Verification items for the finished model (mm, model axes). Face numbers are marked on the shaded views. A direction names the side the tool comes from. Give positions to 0.01 mm unless a question says otherwise; leave off trailing zeros. Loops run counter-clockwise (first coordinate to the right, second up) from the corner with the lowest first, then second, coordinate; pieces in that order, holes last. Notation, with made-up numbers: M 56,7.25 L 67,7.25 A19 cw 67,19.25 Z; hole C 28.25,19.5 d5. An arc over 180 degrees is marked long. Write each question's results on one line, items separated by ' | '. Start each with the question number.
```python
from build123d import *

# Parameters (mm, degrees)
SKETCH1_W           = 50
SKETCH1_H           = 52
BOSS_EXTRUDE1_DEPTH = 61
SKETCH2_W           = 30
SKETCH2_H           = 30
CUT_EXTRUDE1_DEPTH  = 51
CUT_EXTRUDE2_DEPTH  = 75
CUT_EXTRUDE3_DEPTH  = 51
SKETCH6_W           = 50
SKETCH6_H           = 4.1
BOSS_EXTRUDE2_DEPTH = 43
SKETCH8_R           = 11.5
SKETCH8_R_2         = 2
CUT_EXTRUDE4_DEPTH  = 43
BOSS_EXTRUDE3_DEPTH = 3.5
BOSS_EXTRUDE4_DEPTH = 3.5
SKETCH11_R          = 15
CUT_EXTRUDE5_DEPTH  = 98.5
SKETCH12_R          = 15
CUT_EXTRUDE6_DEPTH  = 98.5


with BuildPart() as part:
    # Sketch1 → Boss-Extrude1 (new body)
    with BuildSketch(Plane(origin=(0, 0, 0), x_dir=(1, 0, 0), z_dir=(0, 1, 0))):
        Rectangle(SKETCH1_W, SKETCH1_H)
    extrude(amount=BOSS_EXTRUDE1_DEPTH)

    # Sketch2 → Cut-Extrude1 (cut)
    with BuildSketch(Plane(origin=(0, 61, 0), x_dir=(1, 0, 0), z_dir=(0, 1, 0))):
        Rectangle(SKETCH2_W, SKETCH2_H)
    extrude(amount=-CUT_EXTRUDE1_DEPTH, mode=Mode.SUBTRACT)

    # Sketch3 → Cut-Extrude2 (cut, symmetric)
    with BuildSketch(Plane(origin=(0, 10, 0), x_dir=(1, 0, 0), z_dir=(0, 1, 0))):
        with BuildLine():
            Line((1, 12.5), (1, -12.5))
            ThreePointArc((1, -12.5), (-2, -15.5), (-5, -12.5))
            Line((-5, -12.5), (-5, 12.5))
            ThreePointArc((-5, 12.5), (-2, 15.5), (1, 12.5))
        make_face()
    extrude(amount=CUT_EXTRUDE2_DEPTH, both=True, mode=Mode.SUBTRACT)

    # Sketch5 → Cut-Extrude3 (cut)
    with BuildSketch(Plane(origin=(0, 61, 0), x_dir=(1, 0, 0), z_dir=(0, 1, 0))):
        with BuildLine():
            Line((3.852906206, 15), (3.852906206, -15))
            ThreePointArc((3.852906206, -15), (-2.147093794, -21), (-8.147093794, -15))
            Line((-8.147093794, -15), (-8.147093794, 15))
            ThreePointArc((-8.147093794, 15), (-2.147093794, 21), (3.852906206, 15))
        make_face()
    extrude(amount=-CUT_EXTRUDE3_DEPTH, mode=Mode.SUBTRACT)

    # Sketch6 → Boss-Extrude2 (add)
    with BuildSketch(Plane(origin=(0, 61, 0), x_dir=(1, 0, 0), z_dir=(0, 1, 0))):
        with Locations((0, 23.95)):
            Rectangle(SKETCH6_W, SKETCH6_H)
    extrude(amount=BOSS_EXTRUDE2_DEPTH)

    # Sketch8 → Cut-Extrude4 (cut)
    with BuildSketch(Plane.XY.offset(-21.9)):
        with Locations((-0.305876732, 83.277637399)):
            Circle(SKETCH8_R)
        with Locations((-15.355876732, 68.327637399)):
            Circle(SKETCH8_R_2)
        with Locations((-15.355876732, 98.327637399)):
            Circle(SKETCH8_R_2)
        with Locations((14.644123268, 68.327637399)):
            Circle(SKETCH8_R_2)
        with Locations((14.644123268, 98.327637399)):
            Circle(SKETCH8_R_2)
    extrude(amount=-CUT_EXTRUDE4_DEPTH, mode=Mode.SUBTRACT)

    # Sketch9 → Boss-Extrude3 (add)
    with BuildSketch(Plane.ZY.offset(25)):
        Polygon((-21.9, 61), (2.05, 61), (-21.9, 82.893920103), align=None)
    extrude(amount=-BOSS_EXTRUDE3_DEPTH)

    # Sketch10 → Boss-Extrude4 (add)
    with BuildSketch(Plane(origin=(25, 0, 0), x_dir=(0, 0, -1), z_dir=(1, 0, 0))):
        Polygon((21.9, 61), (-2.05, 61), (21.9, 82.893920103), align=None)
    extrude(amount=-BOSS_EXTRUDE4_DEPTH)

    # Sketch11 → Cut-Extrude5 (cut)
    with BuildSketch(Plane.XY.offset(26)):
        with Locations((0, 36)):
            Circle(SKETCH11_R)
    extrude(amount=-CUT_EXTRUDE5_DEPTH, mode=Mode.SUBTRACT)

    # Sketch12 → Cut-Extrude6 (cut)
    with BuildSketch(Plane(origin=(25, 0, 0), x_dir=(0, 0, -1), z_dir=(1, 0, 0))):
        with Locations((-2.05, 36)):
            Circle(SKETCH12_R)
    extrude(amount=-CUT_EXTRUDE6_DEPTH, mode=Mode.SUBTRACT)


solid = part.part
```
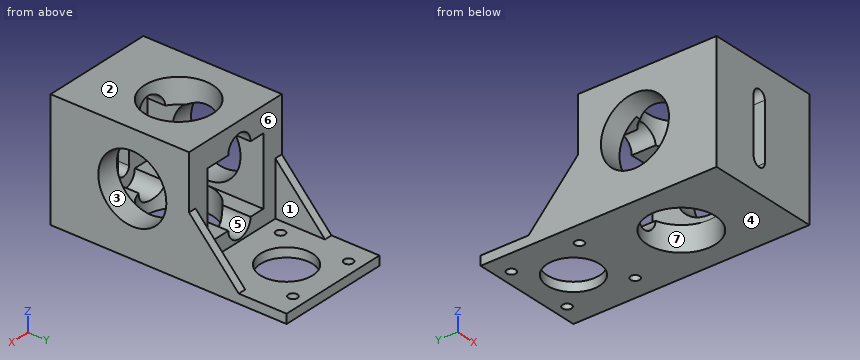
1. Thickness scan on probe 1 along X at (y, z) = (20.5, 0.5); probe 2 along Z at (x, y) = (-5, 63); probe 3 along X at (y, z) = (29, 17.5). Record the ranges inside material, lowest first.
2. Section check D-D, the plane x = 10. Record the boundary of the cut face in (y, z).
3. Release check for a two-part mould opening along Z. For the marked faces 1, 2, 3 and 4 record: released by +Z, released by -Z, zero draft, split by the parting line, or undercut.
4. Section check C-C, the plane x = -19. Record the boundary of the cut face in (y, z).
5. Depth check by flat-ended pin: pin 1 Ø10 at (x, z) = (14.5, 1.5) entering from +Y; pin 2 Ø5 at (x, y) = (14.64, 68.33) entering from +Z. Enter the tip coordinate at first touch or a pass-through.
6. Section check B-B, the plane z = -10.5. Record the boundary of the cut face in (x, y), plus the area to 3 significant figures.
7. Section check A-A, the plane x = -2. Record the boundary of the cut face in (y, z).
8. Set-up check for the marked faces 5, 6 and 7: record each of +Z, -Z, +X, -X, +Y, -Y from which the full face is reachable in a straight line by a thin tool's end or side.
Filled sheet:
1) probe 1: -25 to -15, 15 to 25 | probe 2: -26 to -21.9 | probe 3: -25 to -13.27, 13.27 to 25
2) outline: M 0,-26 L 24.82,-26 L 24.82,-15 L 10,-15 L 10,15 L 24.82,15 L 24.82,26 L 0,26 Z; M 47.18,-26 L 78.17,-26 L 78.17,-21.9 L 61,-21.9 L 61,-15 L 47.18,-15 Z; M 47.18,15 L 61,15 L 61,26 L 47.18,26 Z; M 88.38,-26 L 104,-26 L 104,-21.9 L 88.38,-21.9 Z
3) face 1: zero draft | face 2: released by +Z | face 3: undercut | face 4: released by -Z
4) outline: M 0,-26 L 104,-26 L 104,-21.9 L 61,-21.9 L 61,26 L 0,26 Z; hole C 36,2.05 d30
5) pin 1: y = 61 | pin 2: z = -21.9
6) outline: M -25,0 L -5,0 L -5,10 L -15,10 L -15,27.78 L -25,27.78 Z; M -25,44.22 L -15,44.22 L -15,61 L -21.5,61 L -21.5,72.47 L -25,72.47 Z; M 1,0 L 25,0 L 25,27.78 L 15,27.78 L 15,10 L 1,10 Z; M 15,44.22 L 25,44.22 L 25,72.47 L 21.5,72.47 L 21.5,61 L 15,61 Z | area: 1,210 mm2
7) outline: M 0,-26 L 21.13,-26 L 21.13,-21 L 10,-21 L 10,-15.5 L 0,-15.5 Z; M 0,15.5 L 10,15.5 L 10,21 L 21.13,21 L 21.13,26 L 0,26 Z; M 50.87,-26 L 71.9,-26 L 71.9,-21.9 L 61,-21.9 L 61,-21 L 50.87,-21 Z; M 50.87,21 L 61,21 L 61,26 L 50.87,26 Z; M 94.65,-26 L 104,-26 L 104,-21.9 L 94.65,-21.9 Z
8) face 5: +Y | face 6: +Z, +Y | face 7: +Z, -Z
